Check sheet for the modelled part. Datum: model origin and axes. Units: mm. A direction names the side the tool comes from. Round coordinates to 2 decimals unless told otherwise and drop trailing zeros. Order: outer loops, then holes, each group sorted by start corner. A loop starts at its lowest first (then second) coordinate and runs counter-clockwise, first axis right, second up. Notation, with made-up numbers: (64, 79) -> (121, 79) arc R13 ccw to (121, 83) -> close; hole circle Ø2 at (83, 32.5). An arc over 180 degrees is marked (long way). Answer in a Markdown table with one row per item. Add a question column.
1. Sectioned sample at B-B, the plane y = 126. Record the boundary of the cut face in (x, z).
2. Material ranges on L1, parallel to Y at x = 4.25, z = 6; L2, parallel to Y at x = 5.75, z = 6; L3, parallel to Z at x = 3.75, y = 10, recorded low to high. Write a range as from..to.
3. Sectioned sample at A-A, the plane y = 55. Record the boundary of the cut face in (x, z), then the cut area to 3 significant figures.
4. Depth check by flat-ended pin: P1, Ø9, axis at x = 63.5, y = 85.5, coming from the +Z side; P2, Ø3, axis at x = 50.5, z = 5.5, coming from the +Y side; P3, Ø1, axis at x = 64.5, z = 11, coming from the -Y side. Enter the tip coordinate at first touch or a pass-through.
5. Access from +Z, -Z, +X, -X, +Y, -Y to the whole of each face (thin tool, end or side, straight path). Record for faces 4 (the cylindrical face through (68.895, 102.164, 11.014)), 5 (the flat face through (99, 85, 12)), 6 (the cylindrical face through (4.06, 182.48, 6.33)), 7 (the flat face through (82.62, 162.81, 6.08)).
6. Draft check along Z on faces 1 (the conical face through (96.83, -7.68, 5.87)), 2 (the flat face through (37, 85, 18)), 3 (the cylindrical face through (4.06, 7.78, 4.85)). Enter one of: +Z half, -Z half, draft (parallel to the pull), parting line (faces both ways), or undercut.
```python
from build123d import *

# Parameters (mm, degrees)
SKETCH4_W                    = 122.5
SKETCH4_H                    = 200
BOSS_EXTRUDE1_DEPTH          = 12
CUT_EXTRUDE1_DEPTH           = 12
FILLET1_R                    = 20
FILLET2_R                    = 20
FILLET3_R                    = 10
SKETCH10_R                   = 3.75
BOSS_EXTRUDE3_DEPTH          = 6
F_5_0_5_DIAMETER_HOLE1_D     = 5
F_5_0_5_DIAMETER_HOLE1_DEPTH = 8
F_5_0_5_DIAMETER_HOLE1_TIP   = 1.502151548
F_5_0_5_DIAMETER_HOLE2_D     = 5
F_5_0_5_DIAMETER_HOLE2_DEPTH = 8
F_5_0_5_DIAMETER_HOLE2_TIP   = 1.502151548
SKETCH20_W                   = 93.935697293
SKETCH20_H                   = 45.241593882
SKETCH20_R                   = 2.92490685
SKETCH20_R_2                 = 20.37653906
CUT_EXTRUDE2_DEPTH           = 2
BOSS_EXTRUDE13_START         = 1
SKETCH20_13_R                = 20.37653906
SKETCH20_13_R_2              = 17.641529269
BOSS_EXTRUDE13_DEPTH         = 1
BOSS_EXTRUDE14_START         = 2
SKETCH20_14_R                = 17.641529269
SKETCH20_14_R_2              = 14.663672294
BOSS_EXTRUDE14_DEPTH         = 2
BOSS_EXTRUDE15_START         = 3
SKETCH20_15_R                = 14.663672294
SKETCH20_15_R_2              = 12.74550038
BOSS_EXTRUDE15_DEPTH         = 3
BOSS_EXTRUDE16_START         = 4
SKETCH20_16_R                = 12.74550038
SKETCH20_16_R_2              = 10.504948412
BOSS_EXTRUDE16_DEPTH         = 4
BOSS_EXTRUDE17_START         = 5
SKETCH20_17_R                = 10.504948412
SKETCH20_17_R_2              = 9.019824998
BOSS_EXTRUDE17_DEPTH         = 5
BOSS_EXTRUDE18_START         = 6
SKETCH20_18_R                = 9.019824998
SKETCH20_18_R_2              = 6.837562299
BOSS_EXTRUDE18_DEPTH         = 6
BOSS_EXTRUDE19_START         = 7
SKETCH20_19_R                = 6.837562299
SKETCH20_19_R_2              = 5.911229022
BOSS_EXTRUDE19_DEPTH         = 7
BOSS_EXTRUDE20_START         = 8
SKETCH20_20_R                = 5.911229022
SKETCH20_20_R_2              = 3.525742811
BOSS_EXTRUDE20_DEPTH         = 8
BOSS_EXTRUDE21_START         = 9
SKETCH20_21_R                = 3.525742811
BOSS_EXTRUDE21_DEPTH         = 9
CUT_EXTRUDE3_DEPTH           = 2


with BuildPart() as part:
    # Sketch4 → Boss-Extrude1 (new body)
    with BuildSketch(Plane.XY):
        with Locations((61.25, 100)):
            Rectangle(SKETCH4_W, SKETCH4_H)
    extrude(amount=BOSS_EXTRUDE1_DEPTH)

    # Sketch7 → Cut-Extrude1 (cut)
    with BuildSketch(Plane.XY.offset(12)):
        Polygon((43.985796602, 200), (122.5, 124.415794753), (122.5, 200), align=None)
    extrude(amount=-CUT_EXTRUDE1_DEPTH, mode=Mode.SUBTRACT)

    # Fillet1
    fillet1_edges = [part.edges().sort_by_distance(p)[0] for p in [
        (43.985796602, 200, 6),
    ]]
    fillet(fillet1_edges, radius=FILLET1_R)

    # Fillet2
    fillet2_edges = [part.edges().sort_by_distance(p)[0] for p in [
        (122.5, 124.415794753, 6),
    ]]
    fillet(fillet2_edges, radius=FILLET2_R)

    # Fillet3
    fillet3_edges = [part.edges().sort_by_distance(p)[0] for p in [
        (0, 200, 6),
    ]]
    fillet(fillet3_edges, radius=FILLET3_R)

    # Sketch10 → Boss-Extrude3 (add)
    with BuildSketch(Plane.XZ):
        with Locations(Location((26.25, 6, 0), (0, 0, 90))):
            Circle(SKETCH10_R)
        with Locations(Location((96.25, 6, 0), (0, 0, 90))):
            Circle(SKETCH10_R)
    extrude(amount=BOSS_EXTRUDE3_DEPTH)

    # Boss-Extrude4 cone 1 section (on through the dimple's axis) → Boss-Extrude4 (revolve)
    with BuildSketch(Plane(origin=(26.25, -6, 6), x_dir=(0, 0, 1), z_dir=(1, 0, 0))):
        Polygon((0, 0), (3.75, 0), (0, 1.993910369), align=None)
    revolve(axis=Axis((26.25, -6, 6), (0, -1, 0)))

    # Boss-Extrude4 cone 2 section (on through the dimple's axis) → Boss-Extrude4 cone 2 (revolve)
    with BuildSketch(Plane(origin=(96.25, -6, 6), x_dir=(0, 0, 1), z_dir=(1, 0, 0))):
        Polygon((0, 0), (3.75, 0), (0, 1.993910369), align=None)
    revolve(axis=Axis((96.25, -6, 6), (0, -1, 0)))

    # 5.0 _5_ Diameter Hole1
    with Locations(Plane.ZY):
        with Locations((6, 180)):
            Hole(F_5_0_5_DIAMETER_HOLE1_D / 2, depth=F_5_0_5_DIAMETER_HOLE1_DEPTH)
            with Locations((0, 0, -(F_5_0_5_DIAMETER_HOLE1_DEPTH + F_5_0_5_DIAMETER_HOLE1_TIP / 2))):  # 118° drill point
                Cone(0, F_5_0_5_DIAMETER_HOLE1_D / 2, F_5_0_5_DIAMETER_HOLE1_TIP, mode=Mode.SUBTRACT)

    # 5.0 _5_ Diameter Hole2
    with Locations(Plane.ZY):
        with Locations((6, 10)):
            Hole(F_5_0_5_DIAMETER_HOLE2_D / 2, depth=F_5_0_5_DIAMETER_HOLE2_DEPTH)
            with Locations((0, 0, -(F_5_0_5_DIAMETER_HOLE2_DEPTH + F_5_0_5_DIAMETER_HOLE2_TIP / 2))):  # 118° drill point
                Cone(0, F_5_0_5_DIAMETER_HOLE2_D / 2, F_5_0_5_DIAMETER_HOLE2_TIP, mode=Mode.SUBTRACT)

    # Sketch20 → Cut-Extrude2 (cut)
    with BuildSketch(Plane.XY.offset(12)):
        with Locations((61.361044033, 85.443809719)):
            Rectangle(SKETCH20_W, SKETCH20_H)
        with Locations((67.322275412, 99.697516532)):
            Circle(SKETCH20_R, mode=Mode.SUBTRACT)
        with Locations((35.957607669, 86.013822807)):
            Circle(SKETCH20_R_2, mode=Mode.SUBTRACT)
        with BuildLine():
            add(Edge.make_bspline(
                [(100.146227503, 90.991779166), (102.860896641, 91.009835078), (104.379710297, 89.598437986)],
                knots=[0, 0, 0, 1, 1, 1], degree=2))
            Line((104.379710297, 89.598437986), (106.283646559, 93.405127221))
            add(Edge.make_bspline(
                [(106.283646559, 93.405127221), (100.031028138, 97.418853716), (87.983706785, 92.678641198), (93.854204775, 84.969216201)],
                knots=[0, 0, 0, 0, 1, 1, 1, 1], degree=3))
            add(Edge.make_bspline(
                [(93.854204775, 84.969216201), (98.026734503, 82.096686967), (102.640223397, 80.959953656), (99.911414016, 78.067290297)],
                knots=[0, 0, 0, 0, 1, 1, 1, 1], degree=3))
            add(Edge.make_bspline(
                [(99.911414016, 78.067290297), (98.958240769, 76.804379248), (95.34669814, 76.970567767), (92.89504628, 79.029138763)],
                knots=[0, 0, 0, 0, 1, 1, 1, 1], degree=3))
            Line((92.89504628, 79.029138763), (90.750865037, 75.226412858))
            add(Edge.make_bspline(
                [(90.750865037, 75.226412858), (94.291366297, 72.653681958), (103.101226044, 72.066278851), (105.582611154, 78.774413912)],
                knots=[0, 0, 0, 0, 1, 1, 1, 1], degree=3))
            add(Edge.make_bspline(
                [(105.582611154, 78.774413912), (106.459148582, 82.651459105), (104.591855241, 84.842143282), (99.911414016, 86.581431975)],
                knots=[0, 0, 0, 0, 1, 1, 1, 1], degree=3))
            add(Edge.make_bspline(
                [(99.911414016, 86.581431975), (94.755138706, 89.086680248), (99.08096527, 91.263500215), (100.146227503, 90.991779166)],
                knots=[0, 0, 0, 0, 1, 1, 1, 1], degree=3))
        make_face(mode=Mode.SUBTRACT)
        Polygon((69.26029788, 94.557836932), (61.589041998, 94.557836932), (61.047573723, 90.430188609), (63.683630986, 90.430188609), (61.522270474, 73.953995083), (66.557469092, 73.953995083), align=None, mode=Mode.SUBTRACT)
        with BuildLine():
            add(Edge.make_bspline(
                [(88.590187081, 91.316175115), (90.608809275, 86.564684321), (88.195181264, 78.032608366), (78.503830219, 79.563349573)],
                knots=[0, 0, 0, 0, 1, 1, 1, 1], degree=3))
            add(Edge.make_bspline(
                [(78.503830219, 79.563349573), (75.106377316, 78.083857902), (76.155342876, 76.859276831), (81.296859197, 78.067290297)],
                knots=[0, 0, 0, 0, 1, 1, 1, 1], degree=3))
            add(Edge.make_bspline(
                [(88.126726488, 71.178977426), (90.353172606, 78.355431309), (81.296859197, 78.067290297)],
                knots=[0, 0, 0, 1, 1, 1], degree=2))
            add(Edge.make_bspline(
                [(69.883801172, 68.565818837), (75.441088702, 64.356763635), (85.007837919, 64.558881229), (88.126726488, 71.178977426)],
                knots=[0, 0, 0, 0, 1, 1, 1, 1], degree=3))
            Line((69.883801172, 68.565818837), (73.376875031, 72.316737458))
            add(Edge.make_bspline(
                [(82.35103605, 70.685834384), (79.070911802, 69.329587135), (75.410885248, 70.056928402), (73.376875031, 72.316737458)],
                knots=[0, 0, 0, 0, 1, 1, 1, 1], degree=3))
            add(Edge.make_bspline(
                [(75.937024541, 73.726414789), (86.193415253, 75.228814771), (84.157130117, 71.656945202), (82.35103605, 70.685834384)],
                knots=[0, 0, 0, 0, 1, 1, 1, 1], degree=3))
            add(Edge.make_bspline(
                [(74.817052307, 80.974792322), (72.922567337, 80.410121083), (68.041443, 74.528111598), (75.937024541, 73.726414789)],
                knots=[0, 0, 0, 0, 1, 1, 1, 1], degree=3))
            add(Edge.make_bspline(
                [(85.962196211, 93.951535359), (73.227873525, 98.039311198), (68.565378269, 84.709913686), (74.817052307, 80.974792322)],
                knots=[0, 0, 0, 0, 1, 1, 1, 1], degree=3))
            Line((85.962196211, 93.951535359), (88.126726488, 96.116065636))
            Line((88.126726488, 96.116065636), (91.33219969, 92.910592434))
            Line((91.33219969, 92.910592434), (88.590187081, 91.316175115))
        make_face(mode=Mode.SUBTRACT)
    extrude(amount=-CUT_EXTRUDE2_DEPTH, mode=Mode.SUBTRACT)

    # Sketch20_13 → Boss-Extrude13 (add)
    with BuildSketch(Plane.XY.offset(12).offset(BOSS_EXTRUDE13_START)):
        with Locations((35.957607669, 86.013822807)):
            Circle(SKETCH20_13_R)
        with Locations((37.119063244, 86.818761809)):
            Circle(SKETCH20_13_R_2, mode=Mode.SUBTRACT)
    extrude(amount=-BOSS_EXTRUDE13_DEPTH)

    # Sketch20_14 → Boss-Extrude14 (add)
    with BuildSketch(Plane.XY.offset(12).offset(BOSS_EXTRUDE14_START)):
        with Locations((37.119063244, 86.818761809)):
            Circle(SKETCH20_14_R)
        with Locations((38.428612543, 88.108007113)):
            Circle(SKETCH20_14_R_2, mode=Mode.SUBTRACT)
    extrude(amount=-BOSS_EXTRUDE14_DEPTH)

    # Sketch20_15 → Boss-Extrude15 (add)
    with BuildSketch(Plane.XY.offset(12).offset(BOSS_EXTRUDE15_START)):
        with Locations((38.428612543, 88.108007113)):
            Circle(SKETCH20_15_R)
        with Locations((39.441974393, 88.428639811)):
            Circle(SKETCH20_15_R_2, mode=Mode.SUBTRACT)
    extrude(amount=-BOSS_EXTRUDE15_DEPTH)

    # Sketch20_16 → Boss-Extrude16 (add)
    with BuildSketch(Plane.XY.offset(12).offset(BOSS_EXTRUDE16_START)):
        with Locations((39.441974393, 88.428639811)):
            Circle(SKETCH20_16_R)
        with Locations((40.593265286, 89.13526511)):
            Circle(SKETCH20_16_R_2, mode=Mode.SUBTRACT)
    extrude(amount=-BOSS_EXTRUDE16_DEPTH)

    # Sketch20_17 → Boss-Extrude17 (add)
    with BuildSketch(Plane.XY.offset(12).offset(BOSS_EXTRUDE17_START)):
        with Locations((40.593265286, 89.13526511)):
            Circle(SKETCH20_17_R)
        with Locations((41.099946211, 89.295581459)):
            Circle(SKETCH20_17_R_2, mode=Mode.SUBTRACT)
    extrude(amount=-BOSS_EXTRUDE17_DEPTH)

    # Sketch20_18 → Boss-Extrude18 (add)
    with BuildSketch(Plane.XY.offset(12).offset(BOSS_EXTRUDE18_START)):
        with Locations((41.099946211, 89.295581459)):
            Circle(SKETCH20_18_R)
        with Locations((41.79537959, 90.333458923)):
            Circle(SKETCH20_18_R_2, mode=Mode.SUBTRACT)
    extrude(amount=-BOSS_EXTRUDE18_DEPTH)

    # Sketch20_19 → Boss-Extrude19 (add)
    with BuildSketch(Plane.XY.offset(12).offset(BOSS_EXTRUDE19_START)):
        with Locations(Location((41.79537959, 90.333458923, 0), (0, 0, 180))):
            Circle(SKETCH20_19_R)
        with Locations(Location((42.054997992, 90.430188609, 0), (0, 0, 180))):
            Circle(SKETCH20_19_R_2, mode=Mode.SUBTRACT)
    extrude(amount=-BOSS_EXTRUDE19_DEPTH)

    # Sketch20_20 → Boss-Extrude20 (add)
    with BuildSketch(Plane.XY.offset(12).offset(BOSS_EXTRUDE20_START)):
        with Locations((42.054997992, 90.430188609)):
            Circle(SKETCH20_20_R)
        with Locations((43.134317697, 91.60779599)):
            Circle(SKETCH20_20_R_2, mode=Mode.SUBTRACT)
    extrude(amount=-BOSS_EXTRUDE20_DEPTH)

    # Sketch20_21 → Boss-Extrude21 (add)
    with BuildSketch(Plane.XY.offset(12).offset(BOSS_EXTRUDE21_START)):
        with Locations((43.134317697, 91.60779599)):
            Circle(SKETCH20_21_R)
    extrude(amount=-BOSS_EXTRUDE21_DEPTH)

    # Sketch20_22 → Cut-Extrude3 (cut)
    with BuildSketch(Plane.XY.offset(12)):
        with BuildLine():
            add(Edge.make_bspline(
                [(82.50679273, 90.430188609), (85.773261611, 89.84410729), (84.718395856, 82.229894915), (79.062431364, 83.437020603)],
                knots=[0, 0, 0, 0, 1, 1, 1, 1], degree=3))
            add(Edge.make_bspline(
                [(82.50679273, 90.430188609), (78.139071085, 92.768466485), (74.677374815, 85.246681766), (79.062431364, 83.437020603)],
                knots=[0, 0, 0, 0, 1, 1, 1, 1], degree=3))
        make_face()
    extrude(amount=-CUT_EXTRUDE3_DEPTH, mode=Mode.SUBTRACT)


solid = part.part
```
Answer key:
| question | item | result |
|---|---|---|
| 1 | outline | (0, 0) -> (119.77, 0) -> (119.77, 12) -> (0, 12) -> close |
| 2 | L1 | y = 0..7.5, 12.5..177.5, 182.5..198.18 |
| 2 | L2 | y = 0..7.5, 12.5..177.5, 182.5..199.05 |
| 2 | L3 | z = 0..3.5, 8.5..12 |
| 3 | outline | (0, 0) -> (122.5, 0) -> (122.5, 12) -> (0, 12) -> close |
| 3 | area | 1,470 mm² |
| 4 | P1 | stops at z = 12 |
| 4 | P2 | stops at y = 195.13 |
| 4 | P3 | stops at y = 0 |
| 5 | face 4 | +Z |
| 5 | face 5 | +Z, +X, +Y, -Y |
| 5 | face 6 | -X |
| 5 | face 7 | +Z, -Z, +X, +Y |
| 6 | face 1 | parting line |
| 6 | face 2 | +Z half |
| 6 | face 3 | undercut |
